Design review of the part built by this model. Coordinates are the model's own, in mm. A direction names the side the tool comes from. Give positions to 0.01 mm unless a question says otherwise; leave off trailing zeros. Loops run counter-clockwise (first coordinate to the right, second up) from the corner with the lowest first, then second, coordinate; pieces in that order, holes last. Notation, with made-up numbers: (-2.5, 11.25) - (41.5, 11.25) arc R8 ccw to (41.5, 19.25) - close; hole circle Ø3 at (80, -24.5). An arc over 180 degrees is marked (long way). Write each question's results on one line, items separated by ' | '.
from build123d import *

# Parameters (mm, degrees)
F0_W     = 20
F0_H     = 10
F1_DEPTH = 3
F3_DEPTH = 5
F4_R     = 1.5
F5_DEPTH = 12.5
F6_R     = 3.5
F7_DEPTH = 25


with BuildPart() as f1:
    # F0 (on Top) → F1 (new body)
    with BuildSketch(Plane.XY):
        Rectangle(F0_W, F0_H)
    extrude(amount=F1_DEPTH)

    # F2 (on Front) → F3 (join, symmetric)
    with BuildSketch(Plane.XZ):
        with BuildLine():
            ThreePointArc((5.602103, 18.71108), (0, 5), (-5.602103, 18.71108))
            ThreePointArc((-5.602103, 18.71108), (-6.253786, 20.235457), (-6.498651, 21.875107))
            ThreePointArc((-6.498651, 21.875107), (0, 2), (6.498651, 21.875107))
            ThreePointArc((6.498651, 21.875107), (6.253786, 20.235457), (5.602103, 18.71108))
        make_face()
    extrude(amount=F3_DEPTH, both=True)

    # F4 (on face) → F5 (cut, symmetric)
    with BuildSketch(Plane.XY.offset(3)):
        Circle(F4_R)
    extrude(amount=F5_DEPTH, both=True, mode=Mode.SUBTRACT)

    # F6 (on face) → F7 (cut)
    with BuildSketch(Plane.XY.offset(3)):
        Circle(F6_R)
    extrude(amount=F7_DEPTH, mode=Mode.SUBTRACT)


solid = f1.part
(1) Tool access review of faces 1 (the flat face through (-7, 0, 3)), 2 (the flat face through (-10, 0, 1)), 3 (the flat face through (7, 0, 3)), 4 (the flat face through (10, 0, 1)): name each direction out of +Z, -Z, +X, -X, +Y, -Y from which nothing blocks a thin tool from reaching the whole face with its end or side.
Answers below:
face 1: -X, +Y, -Y | face 2: -Z, -X, +Y, -Y | face 3: +X, +Y, -Y | face 4: -Z, +X, +Y, -Y
(2) Wall thickness on line 1 along Y through (x, z) = (0, 3.8); line 2 along Y through (x, z) = (0, 0.8); line 3 along Z through (x, y) = (-6, 0): over which ranges is each line inside the solid? List them lowest first. Write a range as from..to.
Answers below:
line 1: -5..-3.5, 3.5..5 | line 2: -5..-1.5, 1.5..5 | line 3: 0..3, 3.78..7.71, 18.29..19.51
(3) Take a section at A-A on x = 0. Give the boundary of the cut face in (y, z).
Answers below:
outline: (-5, 0) - (-1.5, 0) - (-1.5, 3) - (-3.5, 3) - (-3.5, 5) - (-5, 5) - close; (1.5, 0) - (5, 0) - (5, 5) - (3.5, 5) - (3.5, 3) - (1.5, 3) - close
(4) Take a section at D-D on x = 6. Give the boundary of the cut face in (y, z).
Answers below:
outline: (-5, 0) - (5, 0) - (5, 3) - (-5, 3) - close; (-5, 3.78) - (5, 3.78) - (5, 7.71) - (-5, 7.71) - close; (-5, 18.29) - (5, 18.29) - (5, 19.51) - (-5, 19.51) - close
(5) Insertion check: P1, Ø0.9, axis at y = 0, z = 2, coming from the -X side; P2, Ø4.5, axis at x = 7, y = -0.5, coming from the +Z side; P3, Ø4, axis at x = 1.5, y = 4, coming from the +Z side; P4, Ø2.5, axis at x = 0, y = 0, coming from the -Z side. Each pin has a flat end and moves straight along its axis. Give the tip position at first contact, or say it passes through.
Answers below:
P1: x = -10 | P2: z = 21.88 | P3: z = 5.81 | P4: through
(6) Take a section at C-C on y = -2.5. Give the boundary of the cut face in (x, z).
Answers below:
outline: (-10, 0) - (10, 0) - (10, 3) - (4.58, 3) arc R11 ccw to (6.5, 21.88) arc R6.5 cw to (5.6, 18.71) arc R8 cw to (2.45, 5.38) - (2.45, 3) - (-2.45, 3) - (-2.45, 5.38) arc R8 cw to (-5.6, 18.71) arc R6.5 cw to (-6.5, 21.88) arc R11 ccw to (-4.58, 3) - (-10, 3) - close
(7) Take a section at B-B on z = 13. Give the boundary of the cut face in (x, y), plus the area to 3 significant figures.
Answers below:
outline: (-11, -5) - (-8, -5) - (-8, 5) - (-11, 5) - close; (8, -5) - (11, -5) - (11, 5) - (8, 5) - close | area: 60.0 mm2
(8) Draft analysis for pull direction Y (two halves, no side actions). For faces 5 (the flat face through (0, -2, 3)), 6 (the flat face through (0, 2, 0)), 7 (the flat face through (0, -5, 4)), state which applies: pulls with the +Y half, pulls with the -Y half, needs draft (parallel to the pull), parting line crosses it, or undercut.
Answers below:
face 5: undercut | face 6: needs draft | face 7: pulls with the -Y half
